Geometry: final body of the model. Coordinates: model frame, mm. Face numbers are marked on the shaded views. A direction names the side the tool comes from. Coordinates: 2 decimals unless noted, no trailing zeros. Order: outer loops, then holes, each group sorted by start corner. A loop starts at its lowest first (then second) coordinate and runs counter-clockwise, first axis right, second up. Notation, with made-up numbers: (12.25, 72.5) - (57.25, 72.5) arc R12 ccw to (57.25, 88.5) - close; hole circle Ø11 at (82, 27.25). An arc over 180 degrees is marked (long way). Use a Markdown table: item, result. Add a question column.
```python
from build123d import *

# Parameters (mm, degrees)
SKETCH1_W           = 59
SKETCH1_H           = 56.6
SKETCH1_W_2         = 50
SKETCH1_H_2         = 47.6
BOSS_EXTRUDE1_DEPTH = 3
BOSS_EXTRUDE2_START = 3
SKETCH1_3_W         = 59
SKETCH1_3_H         = 56.6
SKETCH1_3_W_2       = 50
SKETCH1_3_H_2       = 47.6
BOSS_EXTRUDE2_DEPTH = 52
SKETCH2_W           = 59
SKETCH2_H           = 4.5
BOSS_EXTRUDE3_DEPTH = 4
BOSS_EXTRUDE4_DEPTH = 5
SKETCH4_R           = 1.75
CUT_EXTRUDE1_DEPTH  = 88.639374713
SKETCH5_R           = 3
BOSS_EXTRUDE5_DEPTH = 5
MIRROR1_START       = -34.5
MIRROR1_OUTLINE_R   = 3
MIRROR1_DEPTH       = 5
SKETCH6_W           = 4.242640688
SKETCH6_H           = 4.242640688
BOSS_EXTRUDE6_DEPTH = 5


# Read off the part's stored shape, not the designer's step: Mirror1
with BuildPart() as part:
    # Sketch1 → Boss-Extrude1 (new body)
    # profile 1 of 2: a face of its own
    with BuildSketch(Plane.XY):
        Rectangle(SKETCH1_W, SKETCH1_H)
        Rectangle(SKETCH1_W_2, SKETCH1_H_2, mode=Mode.SUBTRACT)
    # profile 2 of 2: a face of its own
    with BuildSketch(Plane.XY):
        Rectangle(SKETCH1_W_2, SKETCH1_H_2)
    extrude(amount=BOSS_EXTRUDE1_DEPTH)

    # Sketch1<3> → Boss-Extrude2 (add)
    with BuildSketch(Plane.XY.offset(BOSS_EXTRUDE2_START)):
        Rectangle(SKETCH1_3_W, SKETCH1_3_H)
        Rectangle(SKETCH1_3_W_2, SKETCH1_3_H_2, mode=Mode.SUBTRACT)
    extrude(amount=BOSS_EXTRUDE2_DEPTH)

    # Sketch2 → Boss-Extrude3 (add)
    with BuildSketch(Plane.XY.offset(55)):
        with Locations((0, -26.05)):
            Rectangle(SKETCH2_W, SKETCH2_H)
    extrude(amount=BOSS_EXTRUDE3_DEPTH)

    # Sketch3 → Boss-Extrude4 (add)
    with BuildSketch(Plane.XY.offset(59)):
        Polygon((-29.5, -28.3), (-29.5, 16.2), (-25, 16.2), (-25, -23.8), (25, -23.8), (25, 16.2), (29.5, 16.2), (29.5, -28.3), align=None)
    extrude(amount=BOSS_EXTRUDE4_DEPTH)

    # Sketch4 → Cut-Extrude1 (cut, through all)
    with BuildSketch(Plane(origin=(0, -23.8, 0), x_dir=(1, 0, 0), z_dir=(0, 1, 0))):
        with Locations(Location((-27.25, -57, 0), (0, 0, 270))):
            Circle(SKETCH4_R)
        with Locations(Location((27.25, -57, 0), (0, 0, 270))):
            Circle(SKETCH4_R)
    extrude(amount=-CUT_EXTRUDE1_DEPTH, mode=Mode.SUBTRACT)

    # Sketch5 → Boss-Extrude5 (add)
    with BuildSketch(Plane(origin=(29.5, 0, 0), x_dir=(0, 0, -1), z_dir=(1, 0, 0))):
        with Locations(Location((-44, 0, 0), (0, 0, 180))):
            Circle(SKETCH5_R)
        with BuildLine():
            ThreePointArc((-44, -17.67766953), (-26.32233047, 0), (-44, 17.67766953))
            ThreePointArc((-44, 17.67766953), (-46.465060373, 15.212609157), (-44, 12.747548784))
            ThreePointArc((-44, 12.747548784), (-31.252451216, 0), (-44, -12.747548784))
            ThreePointArc((-44, -12.747548784), (-46.465060373, -15.212609157), (-44, -17.67766953))
        make_face()
    extrude(amount=BOSS_EXTRUDE5_DEPTH)

    # Mirror1 outline → Mirror1 (add)
    with BuildSketch(Plane.YZ.offset(MIRROR1_START)):
        with Locations((0, 44)):
            Circle(MIRROR1_OUTLINE_R)
    extrude(amount=MIRROR1_DEPTH)

    # Sketch6 → Boss-Extrude6 (add)
    with BuildSketch(Plane(origin=(34.5, 0, 0), x_dir=(0, 0, -1), z_dir=(1, 0, 0))):
        with Locations((-44, 0)):
            Rectangle(SKETCH6_W, SKETCH6_H)
    extrude(amount=BOSS_EXTRUDE6_DEPTH)


solid = part.part
```
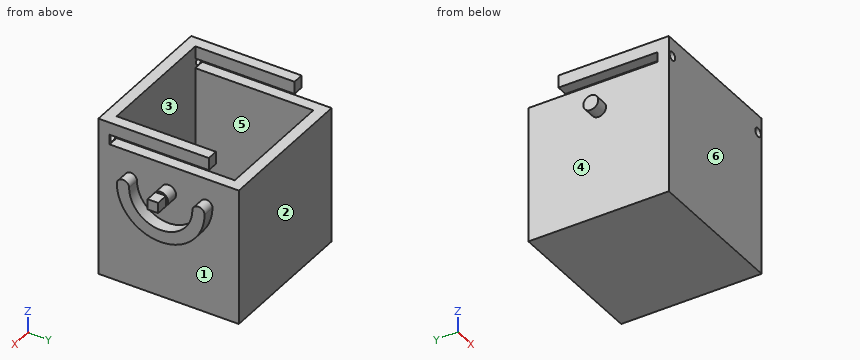
1) Section query C-C (x = -18.5). Return the cut outline in (y, z).
2) Draft query along Y for the marked faces 3, 4, 5 and 6. Return one class per face: released by +Y, released by -Y, zero draft, split by the parting line, or undercut.
3) Line query: line 1 (X direction, y = -25, z = 57); line 2 (Y direction, x = -24.5, z = 4); line 3 (X direction, y = -2, z = 30.5). Output: solid intervals per line, ascending. Write a range as from..to.
4) Section query B-B (x = -27.25). Return the cut outline in (y, z), and give its area (3 significant figures).
5) Access query for the marked faces 1 and 2. Directions: +Z, -Z, +X, -X, +Y, -Y. A direction counts if a zero-diameter tool reaches every point of the face in a straight line with its end or side. Return the directions, or none.
6) Section query A-A (z = 57). Return the cut outline in (x, y).
7) First-contact query: pin 1 (3.5 mm diameter, centred on x = -28, z = 62, fed in from +Y); pin 2 (3.5 mm diameter, centred on x = 37.5, y = -1, fed in from +Z); pin 3 (2 mm diameter, centred on y = -19.5, z = 37.5, fed in from +X); pin 4 (3 mm diameter, centred on x = -19.5, z = 55.5, fed in from +Y). Flat tips, straight axial feed; report the tip coordinate or a pass-through.
8) Section query D-D (y = 9). Return the cut outline in (x, z), and give its area (3 significant figures).
From the geometry:
| question | item | result |
|---|---|---|
| 1 | outline | (-28.3, 0) - (28.3, 0) - (28.3, 55) - (23.8, 55) - (23.8, 3) - (-23.8, 3) - (-23.8, 64) - (-28.3, 64) - close |
| 2 | face 3 | undercut |
| 2 | face 4 | zero draft |
| 2 | face 5 | undercut |
| 2 | face 6 | released by -Y |
| 3 | line 1 | x = -29.5..-29, -25.5..25.5, 29..29.5 |
| 3 | line 2 | y = -28.3..-23.8, 23.8..28.3 |
| 3 | line 3 | x = -29.5..-25, 25..34.5 |
| 4 | outline | (-28.3, 0) - (28.3, 0) - (28.3, 55) - (-23.8, 55) - (-23.8, 55.25) - (-28.3, 55.25) - close; (-28.3, 58.75) - (-23.8, 58.75) - (-23.8, 59) - (16.2, 59) - (16.2, 64) - (-28.3, 64) - close |
| 4 | area | 3,340 mm^2 |
| 5 | face 1 | +X |
| 5 | face 2 | +Z, -Z, +X, -X, +Y |
| 6 | outline | (-29.5, -28.3) - (-29, -28.3) - (-29, -23.8) - (-29.5, -23.8) - close; (-25.5, -28.3) - (25.5, -28.3) - (25.5, -23.8) - (-25.5, -23.8) - close; (29, -28.3) - (29.5, -28.3) - (29.5, -23.8) - (29, -23.8) - close |
| 7 | pin 1 | stops at y = 16.2 |
| 7 | pin 2 | stops at z = 46.12 |
| 7 | pin 3 | stops at x = 29.5 |
| 7 | pin 4 | stops at y = 28.3 |
| 8 | outline | (-29.5, 0) - (29.5, 0) - (29.5, 28.78) - (34.5, 28.78) - (34.5, 34.97) - (29.5, 34.97) - (29.5, 55) - (25, 55) - (25, 3) - (-25, 3) - (-25, 55) - (-29.5, 55) - close; (-29.5, 59) - (-25, 59) - (-25, 64) - (-29.5, 64) - close; (25, 59) - (29.5, 59) - (29.5, 64) - (25, 64) - close |
| 8 | area | 721 mm^2 |
